Part model, mm, in its own coordinate system. A direction names the side the tool comes from. Round coordinates to 2 decimals unless told otherwise and drop trailing zeros. Write each loop counter-clockwise with the first axis right and the second up, starting at its lowest first coordinate (ties: lowest second). Pieces come first, ordered by that corner, then holes. Notation, with made-up numbers: (-12, 47) -> (37, 47) arc R35 ccw to (37, 80) -> close; hole circle Ø11 at (28, 53). An arc over 180 degrees is marked (long way). Use CSV: the item, a comma, the result in double quotes. Start each with the question number.
```python
from build123d import *

# Parameters (mm, degrees)
F0_W     = 30
F0_H     = 70
F1_DEPTH = 1
F3_W     = 22.3
F3_H     = 3.5
F4_DEPTH = 21
F5_DEPTH = 40


with BuildPart() as f1:
    # F0 (on Top) → F1 (new body)
    with BuildSketch(Plane.XY):
        Rectangle(F0_W, F0_H)
    extrude(amount=F1_DEPTH)

    # F3 (on face) → F4 (join)
    with BuildSketch(Plane(origin=(0, 0, 0), x_dir=(1, 0, 0), z_dir=(0, 0, -1))):
        with Locations((0, 7.62)):
            Rectangle(F3_W, F3_H)
        with Locations((0, -7.62)):
            Rectangle(F3_W, F3_H)
    extrude(amount=F4_DEPTH)

    # F3 (on face) → F5 (join)
    with BuildSketch(Plane(origin=(0, 0, 0), x_dir=(1, 0, 0), z_dir=(0, 0, -1))):
        with BuildLine():
            Line((-15, 17.517304), (-15, 33.282696))
            ThreePointArc((-15, 33.282696), (-19.41, 25.4), (-15, 17.517304))
        make_face()
        with BuildLine():
            Line((15, 17.517304), (15, 33.282696))
            ThreePointArc((15, 33.282696), (0.91, 25.4), (15, 17.517304))
        make_face()
        with BuildLine():
            ThreePointArc((-0.91, -25.4), (-5.643779, -17.327438), (-15, -17.517304))
            Line((-15, -17.517304), (-15, -33.282696))
            ThreePointArc((-15, -33.282696), (-5.643779, -33.472562), (-0.91, -25.4))
        make_face()
        with BuildLine():
            ThreePointArc((19.41, -25.4), (18.232562, -20.883779), (15, -17.517304))
            Line((15, -17.517304), (15, -33.282696))
            ThreePointArc((15, -33.282696), (18.232562, -29.916221), (19.41, -25.4))
        make_face()
        with BuildLine():
            Line((-15, -33.282696), (-15, -17.517304))
            ThreePointArc((-15, -17.517304), (-19.41, -25.4), (-15, -33.282696))
        make_face()
        with BuildLine():
            ThreePointArc((-0.91, 25.4), (-5.643779, 33.472562), (-15, 33.282696))
            Line((-15, 33.282696), (-15, 17.517304))
            ThreePointArc((-15, 17.517304), (-5.643779, 17.327438), (-0.91, 25.4))
        make_face()
        with BuildLine():
            ThreePointArc((15, 17.517304), (18.232562, 20.883779), (19.41, 25.4))
            ThreePointArc((19.41, 25.4), (18.232562, 29.916221), (15, 33.282696))
            Line((15, 33.282696), (15, 17.517304))
        make_face()
        with BuildLine():
            Line((15, -33.282696), (15, -17.517304))
            ThreePointArc((15, -17.517304), (0.91, -25.4), (15, -33.282696))
        make_face()
    extrude(amount=F5_DEPTH)


solid = f1.part
```
1. Band-saw the part on C-C (x = 10.16). List the corners of the cut face in (y, z), then the cut area to 3 significant figures.
2. Drill centre lines: line 1 along Y through (x, z) = (0.5, -7); line 2 along X through (y, z) = (25.5, -36); line 3 along Y through (x, z) = (-11, -7). Where is each one in solid material? Low to high. Write a range as [from, to].
3. Pull direction Y, two halves, no side cores. Call faces 6 (the flat face through (0, 0, 0)), 7 (the flat face through (17, -26, 0)): released by +Y, released by -Y, zero draft, split by the parting line, or undercut.
4. Band-saw the part on D-D (y = -21). List the corners of the cut face in (x, z).
5. Which spindle directions (+Z, -Z, +X, -X, +Y, -Y) get a long thin tool onto all of the face, cutting with end or side? Do faces 1 (the flat face through (17, 25, 0)), 2 (the flat face through (-11.15, 8, -10)), 3 (the flat face through (11.15, 8, -10)), 4 (the flat face through (-17, -26, 0)), 5 (the flat face through (0, 8, -21)). Say none if no direction does.
6. Band-saw the part on A-A (z = -27). List the corners of the cut face in (x, y).
7. Flat gauge pins, fed straight in: pin 1 (0.5 mm diameter, centred on y = 7.5, z = 0.5, fed in from -X); pin 2 (6 mm diameter, centred on y = -11, z = -16, fed in from -X); pin 3 (1 mm diameter, centred on x = 3.5, z = -32, fed in from -Y). Where does each tip first touch, or does it go through?
8. Band-saw the part on B-B (z = -19). List the corners of the cut face in (x, y), then the cut area to 3 significant figures.
Answers below:
1,outline,"(-35, 0) -> (-34.65, 0) -> (-34.65, -40) -> (-16.15, -40) -> (-16.15, 0) -> (-9.37, 0) -> (-9.37, -21) -> (-5.87, -21) -> (-5.87, 0) -> (5.87, 0) -> (5.87, -21) -> (9.37, -21) -> (9.37, 0) -> (16.15, 0) -> (16.15, -40) -> (34.65, -40) -> (34.65, 0) -> (35, 0) -> (35, 1) -> (-35, 1) -> close"
1,area,"1,700 mm^2"
2,line 1,"y = [-9.37, -5.87], [5.87, 9.37]"
2,line 2,"x = [-19.41, -0.91], [0.91, 19.41]"
2,line 3,"y = [-34.61, -16.19], [-9.37, -5.87], [5.87, 9.37], [16.19, 34.61]"
3,face 6,"undercut"
3,face 7,"zero draft"
4,outline,"(-18.3, -40) -> (-2.02, -40) -> (-2.02, 0) -> (2.02, 0) -> (2.02, -40) -> (18.3, -40) -> (18.3, 0) -> (15, 0) -> (15, 1) -> (-15, 1) -> (-15, 0) -> (-18.3, 0) -> close"
5,face 1,"+Z, +X, +Y, -Y"
5,face 2,"-Z, -X"
5,face 3,"-Z, +X"
5,face 4,"+Z, -X, +Y, -Y"
5,face 5,"-Z, +X, -X"
6,outline,"(-15, -33.28) arc R9.25 ccw to (-0.91, -25.4) arc R9.25 ccw to (-15, -17.52) arc R9.25 ccw to start; (-15, 17.52) arc R9.25 ccw to (-0.91, 25.4) arc R9.25 ccw to (-15, 33.28) arc R9.25 ccw to start; (15, -33.28) arc R9.25 ccw to (19.41, -25.4) arc R9.25 ccw to (15, -17.52) arc R9.25 ccw (long way) to start; (15, 17.52) arc R9.25 ccw to (19.41, 25.4) arc R9.25 ccw to (15, 33.28) arc R9.25 ccw (long way) to start"
7,pin 1,"stops at x = -15"
7,pin 2,"stops at x = -11.15"
7,pin 3,"stops at y = -32.3"
8,outline,"(-15, -33.28) arc R9.25 ccw to (-0.91, -25.4) arc R9.25 ccw to (-15, -17.52) arc R9.25 ccw to start; (-15, 17.52) arc R9.25 ccw to (-0.91, 25.4) arc R9.25 ccw to (-15, 33.28) arc R9.25 ccw to start; (-11.15, -9.37) -> (11.15, -9.37) -> (11.15, -5.87) -> (-11.15, -5.87) -> close; (-11.15, 5.87) -> (11.15, 5.87) -> (11.15, 9.37) -> (-11.15, 9.37) -> close; (15, -33.28) arc R9.25 ccw to (19.41, -25.4) arc R9.25 ccw to (15, -17.52) arc R9.25 ccw (long way) to start; (15, 17.52) arc R9.25 ccw to (19.41, 25.4) arc R9.25 ccw to (15, 33.28) arc R9.25 ccw (long way) to start"
8,area,"1,230 mm^2"
